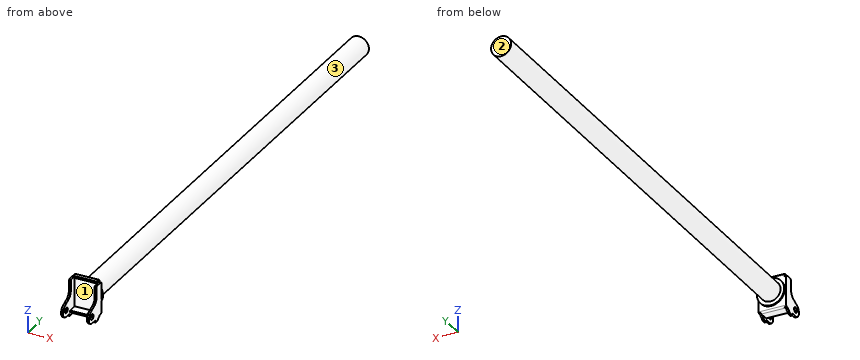
from build123d import *

# Parameters (mm, degrees)
SKETCH1_W           = 35.2425
SKETCH1_H           = 45.085
BOSS_EXTRUDE1_DEPTH = 2.794
SKETCH3_W           = 35.2425
SKETCH3_H           = 7.62
BOSS_EXTRUDE2_DEPTH = 2.794
SKETCH4_W           = 35.2425
SKETCH4_H           = 15.875
BOSS_EXTRUDE3_DEPTH = 2.794
SKETCH5_R           = 3.99415
BOSS_EXTRUDE5_DEPTH = 2.794
SKETCH8_R           = 14.8209
BOSS_EXTRUDE6_DEPTH = 755.65
FILLET1_R           = 2.54


with BuildPart() as part:
    # Sketch1 → Boss-Extrude1 (new body)
    with BuildSketch(Plane(origin=(0, 0, 0), x_dir=(1, 0, 0), z_dir=(0, 1, 0))):
        Rectangle(SKETCH1_W, SKETCH1_H)
    extrude(amount=BOSS_EXTRUDE1_DEPTH)

    # Sketch3 → Boss-Extrude2 (add)
    with BuildSketch(Plane.XY.offset(22.5425)):
        with Locations((0, -1.016)):
            Rectangle(SKETCH3_W, SKETCH3_H)
    extrude(amount=BOSS_EXTRUDE2_DEPTH)

    # Sketch4 → Boss-Extrude3 (add)
    with BuildSketch(Plane(origin=(0, 0, -22.5425), x_dir=(-1, 0, 0), z_dir=(0, 0, -1))):
        with Locations((0, -5.1435)):
            Rectangle(SKETCH4_W, SKETCH4_H)
    extrude(amount=BOSS_EXTRUDE3_DEPTH)

    # Sketch5 → Boss-Extrude5 (add)
    with BuildSketch(Plane.ZY.offset(17.62125)):
        with BuildLine():
            Line((-24.5745, 2.794), (-24.5745, -0.249652205))
            ThreePointArc((-24.5745, -0.249652205), (-24.707295287, -1.060186269), (-25.091795645, -1.785968283))
            Line((-25.091795645, -1.785968283), (-30.3911, -8.763))
            Line((-30.3911, -8.763), (-30.3911, -13.843))
            Line((-30.3911, -13.843), (-26.9875, -13.843))
            Line((-26.9875, -13.843), (-26.9875, -23.3045))
            ThreePointArc((-26.9875, -23.3045), (-19.506235123, -32.571845213), (-8.869629771, -27.213147793))
            Line((-8.869629771, -27.213147793), (-4.188060723, -16.867828085))
            ThreePointArc((-4.188060723, -16.867828085), (-0.439339327, -12.518932794), (5.068277097, -10.8966))
            Line((5.068277097, -10.8966), (19.5707, -10.8966))
            ThreePointArc((19.5707, -10.8966), (21.366751224, -10.152651224), (22.1107, -8.3566))
            Line((22.1107, -8.3566), (22.1107, 0.254))
            ThreePointArc((22.1107, 0.254), (21.366751224, 2.050051224), (19.5707, 2.794))
            Line((19.5707, 2.794), (-24.5745, 2.794))
        make_face()
        with Locations((-17.50695, -23.3045)):
            Circle(SKETCH5_R, mode=Mode.SUBTRACT)
    boss_extrude5 = extrude(amount=BOSS_EXTRUDE5_DEPTH)

    # Mirror1: Boss-Extrude5 across plane
    add(boss_extrude5.mirror(Plane(origin=(0, 0, 0), x_dir=(0, 0, 1), z_dir=(1, 0, 0))))

    # Sketch6 → Revolve1 (revolve)
    with BuildSketch(Plane(origin=(0, 0, 0), x_dir=(0, 0, -1), z_dir=(1, 0, 0))):
        Polygon((0.5588, 2.794), (17.2339, 2.794), (17.2339, 6.1087), (20.5994, 6.1087), (20.5994, 8.1153), (0.5588, 8.1153), align=None)
    revolve(axis=Axis((0, 2.794, -0.5588), (0, 1, 0)))

    # Sketch8 → Boss-Extrude6 (add)
    with BuildSketch(Plane(origin=(0, 8.1153, 0), x_dir=(1, 0, 0), z_dir=(0, 1, 0))):
        Circle(SKETCH8_R)
    extrude(amount=BOSS_EXTRUDE6_DEPTH)

    # Fillet1
    fillet1_edges = [part.edges().sort_by_distance(p)[0] for p in [
        (0, 2.794, -25.3365),
        (0, 2.794, 25.3365),
    ]]
    fillet(fillet1_edges, radius=FILLET1_R)


solid = part.part
Geometry: final body of the model. Coordinates: model frame, mm. Face numbers are marked on the shaded views. Give positions to 0.01 mm unless a question says otherwise; leave off trailing zeros. Order: outer loops, then holes, each group sorted by start corner. A loop starts at its lowest first (then second) coordinate and runs counter-clockwise, first axis right, second up. Notation, with made-up numbers: (61.25, -14.5) -> (105.25, -14.5) arc R12 cw to (105.25, -2.5) -> close; hole circle Ø11 at (70, 54.5). An arc over 180 degrees is marked (long way). Write each question's results on one line, items separated by ' | '.
1) Cut plane B-B (y = 619). Output: boundary loops of the cut face in (x, z).
Geometry says:
outline: circle Ø29.64 at (0, 0)
2) Draft query along X for the marked faces 1, 2 and 3. Return one class per face: released by +X, released by -X, zero draft, split by the parting line, or undercut.
Geometry says:
face 1: undercut | face 2: zero draft | face 3: split by the parting line
3) Cut plane A-A (x = 6.5). Output: boundary loops of the cut face in (y, z), and give its area (3 significant figures).
Geometry says:
outline: (-13.08, -25.34) -> (0.25, -25.34) arc R2.54 ccw to (2.79, -22.8) -> (2.79, -15.91) -> (6.11, -15.91) -> (6.11, -19.52) -> (8.12, -19.52) -> (8.12, -13.32) -> (763.77, -13.32) -> (763.77, 13.32) -> (8.12, 13.32) -> (8.12, 18.4) -> (6.11, 18.4) -> (6.11, 14.8) -> (2.79, 14.8) -> (2.79, 22.8) arc R2.54 ccw to (0.25, 25.34) -> (-4.83, 25.34) -> (-4.83, 22.54) -> (0, 22.54) -> (0, -22.54) -> (-13.08, -22.54) -> close | area: 20,500 mm²
4) First-contact query: pin 1 Ø0.8 at (x, z) = (5.5, -24) entering from -Y; pin 2 Ø12 at (y, z) = (675, 8) entering from -X; pin 3 Ø10 at (x, y) = (14.5, 230) entering from +Z. Flat tips, straight axial feed; report the tip coordinate or a pass-through.
Geometry says:
pin 1: stops at y = -13.08 | pin 2: stops at x = -14.69 | pin 3: stops at z = 11.38
5) Line query: line 1 along Y through (x, z) = (-9.5, -14.5); line 2 along Y through (x, z) = (-14.5, -21.5); line 3 along Y through (x, z) = (-5.5, 2). Output: solid intervals per line, ascending.
Geometry says:
line 1: y = 0 to 2.79, 6.11 to 8.12 | line 2: y = 0 to 2.79 | line 3: y = 0 to 763.77
